Design review of the part built by this model. Coordinates are the model's own, in mm. A direction names the side the tool comes from. Round coordinates to 2 decimals unless told otherwise and drop trailing zeros. Order: outer loops, then holes, each group sorted by start corner. A loop starts at its lowest first (then second) coordinate and runs counter-clockwise, first axis right, second up. Notation, with made-up numbers: (0, 86) - (58, 86) arc R12 cw to (58, 91) - close; hole circle Ø8 at (84, 74). An arc over 180 degrees is marked (long way). Use CSV: the item, a comma, the result in double quotes.
from build123d import *

# Parameters (mm, degrees)
REVOLVE2_ANGLE      = 270
BOSS_EXTRUDE1_DEPTH = 44.45


with BuildPart() as part:
    # Sketch1 → Revolve2 (revolve)
    with BuildSketch(Plane(origin=(0, 0, 0), x_dir=(0, 0, -1), z_dir=(1, 0, 0))):
        Polygon((22.479, 35.498434974), (22.479, 45.023434974), (25.654, 45.023434974), (25.654, 0.573434974), (22.479, 0.573434974), (22.479, 32.323434974), (6.35, 32.323434974), (6.35, 0.573434974), (3.175, 0.573434974), (3.175, 45.023434974), (6.35, 45.023434974), (6.35, 35.498434974), align=None)
    revolve(axis=Axis((0, 45.023434974, 0), (0, -1, 0)), revolution_arc=REVOLVE2_ANGLE)

    # Sketch2 → Boss-Extrude1 (add, through all)
    with BuildSketch(Plane(origin=(0, 45.023434974, 0), x_dir=(1, 0, 0), z_dir=(0, 1, 0))):
        with BuildLine():
            Line((0, 6.35), (0, 3.175))
            Line((0, 3.175), (0, 0))
            Line((0, 0), (-3.175, 0))
            Line((-3.175, 0), (-6.35, 0))
            ThreePointArc((-6.35, 0), (4.490128061, -4.490128061), (0, 6.35))
        make_face()
    extrude(amount=-BOSS_EXTRUDE1_DEPTH)


solid = part.part
1) We need section C-C (z = 12). Give the boundary of the cut face in (x, y), then the cut area to 3 significant figures.
Data:
outline,"(-22.67, 0.57) - (-19.01, 0.57) - (-19.01, 32.32) - (19.01, 32.32) - (19.01, 0.57) - (22.67, 0.57) - (22.67, 45.02) - (19.01, 45.02) - (19.01, 35.5) - (-19.01, 35.5) - (-19.01, 45.02) - (-22.67, 45.02) - close"
area,"447 mm2"
2) For faces 4 (the face through (2, 0.573, 0)), 5 (the face through (0, 23, -4)), 6 (the face through (16.41, 40.33, 15.36)), 7 (the face through (4.636, 16.226, 4.34)), list the 3-axis set-ups (+Z, -Z, +X, -X, +Y, -Y) from which the entire face can be reached by the end or side of a thin tool; tool diameter is ignored.
Data:
face 4,"+Z, -Z, +X, -X, -Y"
face 5,"-Z, -X, +Y, -Y"
face 6,"+Y"
face 7,"-Y"
3) We need section A-A (y = 40). Give the boundary of the cut face in (x, z), then the cut area to 3 significant figures.
Data:
outline,"(-25.65, 0) - (-22.48, 0) arc R22.48 cw (long way) to (0, -22.48) - (0, -25.65) arc R25.65 ccw (long way) to start; (-6.35, 0) - (0, 0) - (0, -6.35) arc R6.35 ccw (long way) to start"
area,"455 mm2"
4) To check wall thickness, follow L1, parallel to Z at x = 2.5, y = 24.5; L2, parallel to Y at x = -16.5, z = 15; L3, parallel to Z at x = -3, y = 39. State the ranges of each line that lie inside material, in increasing order. Write a range as from..to.
Data:
L1,"z = -25.53..-22.34, -5.84..5.84, 22.34..25.53"
L2,"y = 32.32..35.5"
L3,"z = 0..5.6, 22.28..25.48"
5) We need section B-B (x = 21.5). Give the boundary of the cut face in (y, z), then the cut area to 3 significant figures.
Data:
outline,"(0.57, -14) - (45.02, -14) - (45.02, -6.56) - (35.5, -6.56) - (35.5, 6.56) - (45.02, 6.56) - (45.02, 14) - (0.57, 14) - (0.57, 6.56) - (32.32, 6.56) - (32.32, -6.56) - (0.57, -6.56) - close"
area,"703 mm2"
6) Insertion check: pin 1 Ø2 at (y, z) = (19, -9) entering from +X; pin 2 Ø1.5 at (x, z) = (-11, 17.5) entering from +Y; pin 3 Ø1.5 at (x, y) = (-7.5, 20) entering from +Z; pin 4 Ø10 at (x, z) = (-5.5, -15) entering from +Y. Each pin has a flat end and moves straight along its axis. Give the tip position at first contact, or say it passes through.
Data:
pin 1,"stops at x = 24.37"
pin 2,"stops at y = 35.5"
pin 3,"stops at z = 24.75"
pin 4,"passes through"
7) The part is to be moulded in two halves that separate along Z. For faces 1 (the face through (5, 35.498, 5)), 2 (the face through (-4, 23, 0)), 3 (the face through (15, 0.573, 17)), say which applies: +Z half, -Z half, draft (parallel to the pull), parting line (faces both ways), or undercut.
Data:
face 1,"undercut"
face 2,"-Z half"
face 3,"draft"
